```python
from build123d import *

# Parameters (mm, degrees)
ESBO_O1_R                = 1.5
RESSALTO_EXTRUS_O1_DEPTH = 1.5


with BuildPart() as part:
    # Esboço1 → Ressalto-extrusão1 (new body)
    with BuildSketch(Plane(origin=(0, 0, 0), x_dir=(1, 0, 0), z_dir=(0, 1, 0))):
        with BuildLine():
            Line((-19, 25), (-19, -12.038750305))
            ThreePointArc((-19, -12.038750305), (-18.802606473, -12.905127766), (-18.249390095, -13.600487924))
            Line((-18.249390095, -13.600487924), (-4.547827976, -24.561737619))
            ThreePointArc((-4.547827976, -24.561737619), (-3.960451764, -24.887256638), (-3.298437881, -25))
            Line((-3.298437881, -25), (4.712, -25))
            Line((4.712, -25), (11.645934077, -25))
            ThreePointArc((11.645934077, -25), (12.767191696, -24.656134461), (13.502887459, -23.742781353))
            Line((13.502887459, -23.742781353), (20.856953382, -5.357616546))
            ThreePointArc((20.856953382, -5.357616546), (20.963912773, -4.993050235), (21, -4.614835193))
            Line((21, -4.614835193), (21, 2.171572875))
            ThreePointArc((21, 2.171572875), (20.847759065, 2.93693974), (20.414213562, 3.585786438))
            Line((20.414213562, 3.585786438), (19.585786438, 4.414213562))
            ThreePointArc((19.585786438, 4.414213562), (19.152240935, 5.06306026), (19, 5.828427125))
            Line((19, 5.828427125), (19, 25))
            Line((19, 25), (-19, 25))
        make_face()
        with Locations(Location((7, -21, 0), (0, 0, 270))):
            Circle(ESBO_O1_R, mode=Mode.SUBTRACT)
        with Locations(Location((9.5, 0, 0), (0, 0, 270))):
            Circle(ESBO_O1_R, mode=Mode.SUBTRACT)
        with Locations(Location((16, -2, 0), (0, 0, 270))):
            Circle(ESBO_O1_R, mode=Mode.SUBTRACT)
        with Locations(Location((-5.5, 0, 0), (0, 0, 270))):
            Circle(ESBO_O1_R, mode=Mode.SUBTRACT)
    extrude(amount=RESSALTO_EXTRUS_O1_DEPTH)


solid = part.part
```
Can you work these out from the model? Positions are in its coordinate system, mm. A direction names the side the tool comes from. Round coordinates to 2 decimals unless told otherwise and drop trailing zeros. Order: outer loops, then holes, each group sorted by start corner. A loop starts at its lowest first (then second) coordinate and runs counter-clockwise, first axis right, second up.
(1) We'd pull the mould along Z, two halves only. Please class faces 1 (the face through (-11.5, 0.7, 19)), 2 (the face through (19.156, 0.74, -5.053)), 3 (the face through (8, 1, 0)): +Z half, -Z half, draft (parallel to the pull), parting line (faces both ways), or undercut.
Results are:
face 1: +Z half
face 2: -Z half
face 3: undercut
(2) If I drill on L1, parallel to X at y = 1, z = 0; L2, parallel to X at y = 1.2, z = 2; L3, parallel to X at y = 1.4, z = -21, over which ranges is the centre line in solid material (lowest first)?
Results are:
L1: x = -19 to -7, -4 to 8, 11 to 21
L2: x = -19 to 14.5, 17.5 to 21
L3: x = -19 to 19
(3) If we section it at B-B (x = -5.5): Please give me the cut outline in (y, z), plus the area to 3 significant figures.
Results are:
outline: (0, -25) - (1.5, -25) - (1.5, -1.5) - (0, -1.5) - close; (0, 1.5) - (1.5, 1.5) - (1.5, 23.8) - (0, 23.8) - close
area: 68.7 mm2
(4) If we section it at D-D (z = -0.5): Please give me the cut outline in (x, y).
Results are:
outline: (-19, 0) - (-6.91, 0) - (-6.91, 1.5) - (-19, 1.5) - close; (-4.09, 0) - (8.09, 0) - (8.09, 1.5) - (-4.09, 1.5) - close; (10.91, 0) - (21, 0) - (21, 1.5) - (10.91, 1.5) - close
(5) If we section it at A-A (z = 21): Please give me the cut outline in (x, y), plus the area to 3 significant figures.
Results are:
outline: (-9, 0) - (5.5, 0) - (5.5, 1.5) - (-9, 1.5) - close; (8.5, 0) - (14.6, 0) - (14.6, 1.5) - (8.5, 1.5) - close
area: 30.9 mm2
(6) If we section it at C-C (y = 0.8): Please give me the cut outline in (x, z).
Results are:
outline: (-19, -25) - (19, -25) - (19, -5.83) arc R2 cw to (19.59, -4.41) - (20.41, -3.59) arc R2 ccw to (21, -2.17) - (21, 4.61) arc R2 ccw to (20.86, 5.36) - (13.5, 23.74) arc R2 ccw to (11.65, 25) - (-3.3, 25) arc R2 ccw to (-4.55, 24.56) - (-18.25, 13.6) arc R2 ccw to (-19, 12.04) - close; hole circle Ø3 at (-5.5, 0); hole circle Ø3 at (7, 21); hole circle Ø3 at (9.5, 0); hole circle Ø3 at (16, 2)
(7) On a 3-axis mill with a long thin cutter (end or side, diameter ignored), from which of +Z, -Z, +X, -X, +Y, -Y can I reach the whole of each face in a straight line? I mean faces 4 (the face through (19, 1, -15)), 5 (the face through (21, 1, 1)). Say none if no direction works.
Results are:
face 4: -Z, +X, +Y, -Y
face 5: +Z, -Z, +X, +Y, -Y
